from build123d import *

# Parameters (mm, degrees)
CYLINDER_R                  = 9.7
CYLINDER_DEPTH              = 100
CYLINDER_ROLL_ANGLE         = -90
CYLINDER_PITCH_ANGLE        = -18.434967
CYLINDER_PLACEMENT_ANGLE    = 18.434967
CYLINDER001_R               = 8
CYLINDER001_DEPTH           = 100
CYLINDER001_ROLL_ANGLE      = -90
CYLINDER001_PITCH_ANGLE     = 45
CYLINDER001_PLACEMENT_ANGLE = -45
REVOLUTION_ANGLE            = -180
SKETCH005_R                 = 6
PAD001_DEPTH                = 8
PAD001_DEPTH_BACK           = 25
PAD002_DEPTH                = 75
SKETCH_R                    = 40
PAD_DEPTH                   = 8
POCKET_DEPTH                = 6.5


with BuildPart() as cylinder:
    # Cylinder → Cylinder (new body)
    with BuildSketch(Plane.XY):
        Circle(CYLINDER_R)
    extrude(amount=CYLINDER_DEPTH)


with BuildPart() as cylinder_1:
    # Cylinder roll: moved
    add(cylinder.part.rotate(Axis((0, 0, 0), (1, 0, 0)), CYLINDER_ROLL_ANGLE))


with BuildPart() as cylinder_2:
    # Cylinder pitch: moved
    add(cylinder_1.part.rotate(Axis((0, 0, 0), (0, 1, 0)), CYLINDER_PITCH_ANGLE))


with BuildPart() as cylinder_3:
    # Cylinder placement: moved
    add(cylinder_2.part.moved(Location((0, 0, -20))).rotate(Axis((0, 0, -20), (0, 0, 1)), CYLINDER_PLACEMENT_ANGLE))


with BuildPart() as fusion001:
    # Cylinder001 → Cylinder001 (new body)
    with BuildSketch(Plane.XY):
        Circle(CYLINDER001_R)
    extrude(amount=CYLINDER001_DEPTH)


with BuildPart() as fusion001_1:
    # Cylinder001 roll: moved
    add(fusion001.part.rotate(Axis((0, 0, 0), (1, 0, 0)), CYLINDER001_ROLL_ANGLE))


with BuildPart() as fusion001_2:
    # Cylinder001 pitch: moved
    add(fusion001_1.part.rotate(Axis((0, 0, 0), (0, 1, 0)), CYLINDER001_PITCH_ANGLE))


with BuildPart() as fusion001_3:
    # Cylinder001 placement: moved
    add(fusion001_2.part.moved(Location((0, 0, -20))).rotate(Axis((0, 0, -20), (0, 0, 1)), CYLINDER001_PLACEMENT_ANGLE))

    # Fusion001: union Cylinder
    add(cylinder_3.part)


with BuildPart() as revolution:
    # Sketch004 → Revolution (revolve)
    with BuildSketch(Plane.YZ):
        with BuildLine():
            Line((48.363934, -6.363988), (46.242623, -4.242658))
            ThreePointArc((46.242623, -4.242658), (47.543272, -2.296112), (48, 0))
            Line((48, 0), (51, 0))
            ThreePointArc((48.363934, -6.363988), (50.314909, -3.444168), (51, 0))
        make_face()
    revolve(axis=Axis((0, 0, 0), (0, 0, 1)), revolution_arc=REVOLUTION_ANGLE)


with BuildPart() as pad001:
    # Sketch005 → Pad001 (new body, two sides)
    with BuildSketch(Plane.XY) as pad001_sk:
        with Locations((-16.492364, 50.758278)):
            Circle(SKETCH005_R)
        with Locations((35.894688, 35.894688)):
            Circle(SKETCH005_R)
    extrude(amount=PAD001_DEPTH)
    extrude(pad001_sk.sketch, amount=-PAD001_DEPTH_BACK)


with BuildPart() as pad002:
    # Sketch006 → Pad002 (new body)
    with BuildSketch(Plane.YZ):
        with BuildLine():
            Line((48.363934, -6.363988), (46.242623, -4.242658))
            ThreePointArc((46.242623, -4.242658), (47.543272, -2.296112), (48, 0))
            Line((48, 0), (51, 0))
            ThreePointArc((48.363934, -6.363988), (50.314909, -3.444168), (51, 0))
        make_face()
    extrude(amount=-PAD002_DEPTH)


with BuildPart() as cut:
    # Sketch → Pad (new body)
    with BuildSketch(Plane.XY):
        with BuildLine():
            ThreePointArc((-46.914816, -20), (42.549971, -28.115832), (0, 51))
            Line((-75, 51), (0, 51))
            ThreePointArc((-75, 51), (-81.690324, 30.60121), (-71.383422, 11.769352))
            ThreePointArc((-46.914816, -20), (-57.126294, -2.557354), (-71.383422, 11.769352))
        make_face()
        Circle(SKETCH_R, mode=Mode.SUBTRACT)
    extrude(amount=PAD_DEPTH)

    # Sketch001 → Pocket (cut)
    with BuildSketch(Plane(origin=(0, 0, 0), x_dir=(1, 0, 0), z_dir=(0, 0, -1))):
        with BuildLine():
            Line((-146.216, -48), (0, -48))
            ThreePointArc((0, -48), (48, 0), (0, 48))
            Line((0, 48), (-146.216, 48))
            Line((-146.216, -48), (-146.216, 48))
        make_face()
    extrude(amount=-POCKET_DEPTH, mode=Mode.SUBTRACT)

    # Fusion: union Revolution, Pad001, Pad002
    add(revolution.part)
    add(pad001.part)
    add(pad002.part)

    # Cut: cut Fusion001
    add(fusion001_3.part, mode=Mode.SUBTRACT)


solid = cut.part
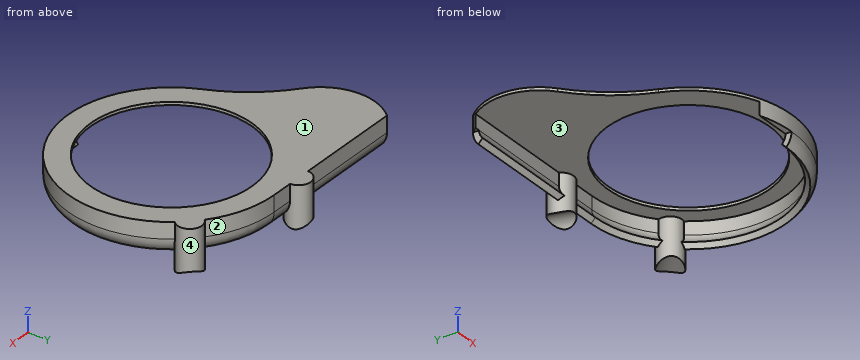
Could you check a few things on this model? Use its own coordinates, in mm. Face numbers are marked on the shaded views. Coordinates: 2 decimals unless noted, no trailing zeros. Order: outer loops, then holes, each group sorted by start corner. A loop starts at its lowest first (then second) coordinate and runs counter-clockwise, first axis right, second up. Notation, with made-up numbers: (-7.5, -33) -> (23.5, -33) arc R7 ccw to (23.5, -27) -> close; hole circle Ø8 at (2, 74). An arc over 180 degrees is marked (long way). One line per item, written item: value. Start each with the question number.
1) I'm going to push flat-ended pins straight in: pin 1 (2.5 mm diameter, centred on y = 47.5, z = -5, fed in from -X); pin 2 (1.4 mm diameter, centred on y = -47.5, z = -3.5, fed in from -X); pin 3 (2 mm diameter, centred on y = 26, z = -9, fed in from +X); pin 4 (1 mm diameter, centred on x = -49, z = 5.5, fed in from +Y). Where does each tip first touch, or does it pass through?
2) Imagine slicing it at B-B on z = 1.5. List the corners of the cut face in (x, y) for me, plus the area to 3 significant figures.
3) If I drill on L1, parallel to Z at x = -41, y = -14; L2, parallel to X at y = 0, z = 6.8; L3, parallel to Z at x = 45.5, y = -10.5, over which ranges is the centre line in solid material (lowest first)? Write a range as [from, to].
4) Imagine slicing it at C-C on x = -55. List the corners of the cut face in (y, z) for me, plus the area to 3 significant figures.
5) We'd pull the mould along Y, two halves only. Please class the marked faces 1, 2, 3 and 4: +Y half, -Y half, draft (parallel to the pull), parting line (faces both ways), or undercut.
6) Imagine slicing it at A-A on y = 0. List the corners of the cut face in (x, z) for me.
Answer list:
1. pin 1: stops at x = -75
1. pin 2: stops at x = 0
1. pin 3: passes through
1. pin 4: stops at y = 51
2. outline: (-77.31, 48) -> (-21.82, 48) arc R6 ccw to (-11.16, 48) -> (0, 48) arc R48 cw to (30.09, 37.4) arc R6 ccw to (37.4, 30.09) arc R48 cw to (0, -48) -> (-17.23, -48) arc R51 ccw to (40.05, 31.57) arc R6 ccw (long way) to (31.57, 40.05) arc R51 ccw to (0, 51) -> (-10.5, 51) arc R6 ccw to (-22.49, 51) -> (-75, 51) arc R27 ccw to start
2. area: 887 mm2
3. L1: z = [6.5, 8]
3. L2: x = [-59.18, -40], [40, 51]
3. L3: z = [-4.7, -3.73], [6.5, 8]
4. outline: (-5.45, 6.5) -> (48, 6.5) -> (48, 0) arc R6 cw to (46.24, -4.24) -> (48.36, -6.36) arc R9 ccw to (51, 0) -> (51, 8) -> (-5.45, 8) -> close
4. area: 122 mm2
5. face 1: draft
5. face 2: +Y half
5. face 3: undercut
5. face 4: undercut
6. outline: (-59.18, 6.5) -> (-40, 6.5) -> (-40, 8) -> (-59.18, 8) -> close; (40, 6.5) -> (48, 6.5) -> (48, 0) arc R6 cw to (46.24, -4.24) -> (48.36, -6.36) arc R9 ccw to (51, 0) -> (51, 8) -> (40, 8) -> close
